Autodesk Inventor part; units mm, degrees
ref_plane "YZ Plane" through (0, 0, 0) normal (1, 0, 0) x (0, 1, 0)
ref_plane "XZ Plane" through (0, 0, 0) normal (0, 1, 0) x (-1, 0, 0)
ref_plane "XY Plane" through (0, 0, 0) normal (0, 0, 1) x (1, 0, 0)
sketch "Sketch1" plane through (0, 0, 0) normal (0, 1, 0) x (-1, 0, 0)
  line L0 (0, 0) -> (50, 0)
  line L1 (50, 0) -> (50, -120)
  line L2 (50, -120) -> (0, -120)
  line L3 (0, -120) -> (0, 0)
  circle A0 centre (35, -31.5) radius 5.1
  circle A1 centre (25, -95) radius 12.5
  arc A2 (0, -95) -> (50, -95) centre (25, -95) ccw
  line L4 (45, 0) -> (34, 0)
  line L5 (34, 0) -> (34, -2)
  line L6 (34, -2) -> (45, -2)
  line L7 (45, -2) -> (45, 0)
  line L8 (16, -2) -> (5, -2)
  line L9 (5, -2) -> (5, 0)
  line L10 (5, 0) -> (16, 0)
  line L11 (16, 0) -> (16, -2)
  line L12 (50, -95) -> (0, -95) construction
  circle A3 centre (15, -31.5) radius 5.1
  dimension "d0" = 10.2
  dimension "d1" = 25
  dimension "d2" = 2
  dimension "d3" = 2
  dimension "d6" = 5
  dimension "d7" = 11
  dimension "d8" = 5
  dimension "d9" = 11
  dimension "d10" = 50
  dimension "d12" = 25
  dimension "d13" = 120
  dimension "d14" = 31.5
  dimension "d16" = 10.2
  dimension "d17" = 31.5
  dimension "d18" = 20
  dimension "d19" = 15
extrude "Plate2" add sketch "Sketch1" along normal blind 2 contours L0 L9 L8 L11 L5 L6 L7 L1 A2 L3
equation "\"d7\" = d9"
equation "\"d12\" = 0.5 * d10"
equation "\"d17\" = d14"
equation "\"d19\" = -0.5 * d18 + 0.5 * d10"
equation "\"d20\" = Thickness"
equation "\"BendRadius\" = Thickness"
equation "\"BendReliefWidth\" = Thickness"
equation "\"BendReliefDepth\" = 0.5 * Thickness"
equation "\"CornerReliefSize\" = 4 * Thickness"
equation "\"MinimumRemnant\" = 2 * Thickness"
equation "\"TransitionRadius\" = BendRadius"
equation "\"JacobiRadiusSize\" = BendRadius"
equation "\"GapSize\" = Thickness"
properties part number "side_beslag"
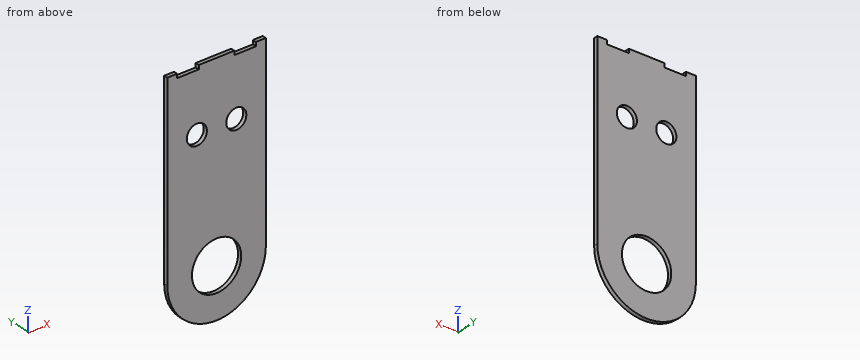
For this review, take the finished solid that the model builds, in its own axes (mm). Give positions to 0.01 mm unless a question says otherwise; leave off trailing zeros. Loops run counter-clockwise (first coordinate to the right, second up) from the corner with the lowest first, then second, coordinate; pieces in that order, holes last. Notation, with made-up numbers: M -31.75,-36.75 L 5.25,-36.75 A18 cw 5.25,-5.75 Z; hole C 46,-37.75 d11. An arc over 180 degrees is marked long. One line per item, written item: value. Start each with the question number.
Q1. For L1, parallel to Z at x = -35, y = 0.4; L2, parallel to Z at x = -33, y = 0.75; L3, parallel to Z at x = -26, y = 0.4, list the stretches that pass through material, from the lowest coordinate up.
Q2. Add section C-C (y = 0.85). Give the boundary of the cut face in (x, z).
Q3. Add section B-B (x = -25). Give the boundary of the cut face in (y, z), and give its area (3 significant figures).
Q4. Clearance check with flat-ended pins moving along their axes: pin 1 Ø1 at (x, y) = (-40.5, 2) entering from +Z; pin 2 Ø9 at (x, z) = (-15, -31.5) entering from -Y; pin 3 Ø1 at (x, y) = (-16, 0) entering from -Z. State where each tip first meets the part, or that it passes through.
Q5. Add section A-A (z = -31.5). Give the boundary of the cut face in (x, y).
Q6. Add section D-D (x = -35.5). Give the boundary of the cut face in (y, z), and give its area (3 significant figures).
Reply:
1. L1: -117.91 to -102.5, -87.5 to -36.6, -26.4 to -2
1. L2: -118.69 to -104.6, -85.4 to -36.19, -26.81 to 0
1. L3: -119.98 to -107.46, -82.54 to 0
2. outline: M -50,-95 A25 ccw 0,-95 L 0,0 L -5,0 L -5,-2 L -16,-2 L -16,0 L -34,0 L -34,-2 L -45,-2 L -45,0 L -50,0 Z; hole C -35,-31.5 d10.2; hole C -25,-95 d25; hole C -15,-31.5 d10.2
3. outline: M 0,-120 L 2,-120 L 2,-107.5 L 0,-107.5 Z; M 0,-82.5 L 2,-82.5 L 2,0 L 0,0 Z
3. area: 190 mm²
4. pin 1: z = -2
4. pin 2: through
4. pin 3: z = -118.51
5. outline: M -50,0 L -40.1,0 L -40.1,2 L -50,2 Z; M -29.9,0 L -20.1,0 L -20.1,2 L -29.9,2 Z; M -9.9,0 L 0,0 L 0,2 L -9.9,2 Z
6. outline: M 0,-117.69 L 2,-117.69 L 2,-101.78 L 0,-101.78 Z; M 0,-88.22 L 2,-88.22 L 2,-36.58 L 0,-36.58 Z; M 0,-26.42 L 2,-26.42 L 2,-2 L 0,-2 Z
6. area: 184 mm²
